For this review, take the finished solid that the model builds, in its own axes (mm). Face numbers are marked on the shaded views. Round coordinates to 2 decimals unless told otherwise and drop trailing zeros. Loops run counter-clockwise (first coordinate to the right, second up) from the corner with the lowest first, then second, coordinate; pieces in that order, holes last. Notation, with made-up numbers: (-10.5, 11) -> (6.5, 11) arc R17 ccw to (6.5, 24) -> close; hole circle Ø8 at (71.25, 10.25). An arc over 180 degrees is marked (long way). Use one line per item in the form item = value. Start each with the question number.
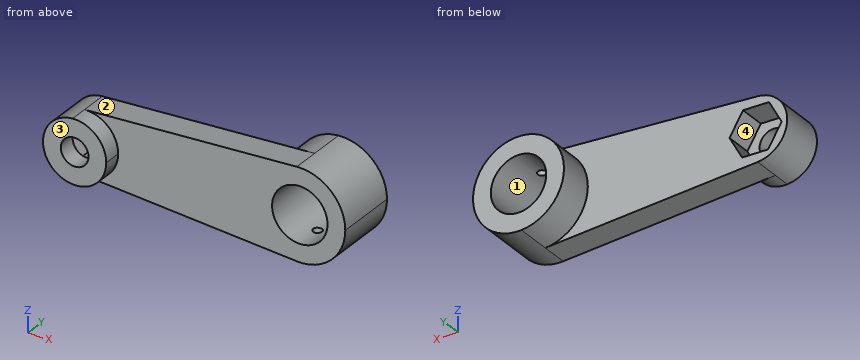
from build123d import *

# Parameters (mm, degrees)
F0_R     = 4.953
F1_DEPTH = 15.875
F0_R_2   = 9.906
F2_DEPTH = 9.525
F3_DEPTH = 12.7
F5_DEPTH = 9.525
F6_R     = 1.5875
F7_DEPTH = 15.875


with BuildPart() as f1:
    # F0 (on Front) → F1 (new body)
    with BuildSketch(Plane.XZ):
        with BuildLine():
            ThreePointArc((-0.734695, -11.279097), (7.72831, -8.248093), (11.303, 0))
            ThreePointArc((11.303, 0), (7.72831, 8.248093), (-0.734695, 11.279097))
            ThreePointArc((-0.734695, 11.279097), (-11.303, 0), (-0.734695, -11.279097))
        make_face()
        Circle(F0_R, mode=Mode.SUBTRACT)
    extrude(amount=F1_DEPTH)

    # F0 (on Front) → F2 (join)
    with BuildSketch(Plane.XZ):
        with BuildLine():
            ThreePointArc((-0.734695, -11.279097), (7.72831, -8.248093), (11.303, 0))
            ThreePointArc((11.303, 0), (7.72831, 8.248093), (-0.734695, 11.279097))
            ThreePointArc((-0.734695, 11.279097), (-11.303, 0), (-0.734695, -11.279097))
        make_face()
        Circle(F0_R, mode=Mode.SUBTRACT)
        with BuildLine():
            ThreePointArc((-0.734695, 11.279097), (7.72831, 8.248093), (11.303, 0))
            ThreePointArc((11.303, 0), (7.72831, -8.248093), (-0.734695, -11.279097))
            Line((-0.734695, -11.279097), (75.14336, -16.221623))
            ThreePointArc((75.14336, -16.221623), (59.944, 0), (75.14336, 16.221623))
            Line((75.14336, 16.221623), (-0.734695, 11.279097))
        make_face()
        with BuildLine():
            ThreePointArc((92.456, 0), (87.314873, 11.862425), (75.14336, 16.221623))
            ThreePointArc((75.14336, 16.221623), (59.944, 0), (75.14336, -16.221623))
            ThreePointArc((75.14336, -16.221623), (87.314873, -11.862425), (92.456, 0))
        make_face()
        with Locations((76.2, 0)):
            Circle(F0_R_2, mode=Mode.SUBTRACT)
    extrude(amount=F2_DEPTH)

    # F0 (on Front) → F3 (join)
    with BuildSketch(Plane.XZ):
        with BuildLine():
            ThreePointArc((92.456, 0), (87.314873, 11.862425), (75.14336, 16.221623))
            ThreePointArc((75.14336, 16.221623), (59.944, 0), (75.14336, -16.221623))
            ThreePointArc((75.14336, -16.221623), (87.314873, -11.862425), (92.456, 0))
        make_face()
        with Locations((76.2, 0)):
            Circle(F0_R_2, mode=Mode.SUBTRACT)
    extrude(amount=-F3_DEPTH)

    # F4 (on Front) → F5 (cut)
    with BuildSketch(Plane.XZ):
        Polygon((-4.819749, 7.967741), (-9.310141, -0.190155), (-4.490392, -8.157896), (4.819749, -7.967741), (9.310141, 0.190155), (4.490392, 8.157896), align=None)
    extrude(amount=F5_DEPTH, mode=Mode.SUBTRACT)

    # F6 (on Top) → F7 (cut, symmetric)
    with BuildSketch(Plane.XY):
        with Locations((76.223016, 0)):
            Circle(F6_R)
    extrude(amount=F7_DEPTH, both=True, mode=Mode.SUBTRACT)


solid = f1.part
Item 1: Take a section at B-B on y = -5.25. Give the boundary of the cut face in (x, z), plus the area to 3 significant figures.
Item 2: Draft analysis for pull direction Z (two halves, no side actions). For the marked faces 1, 2, 3 and 4, state which applies: +Z half, -Z half, draft (parallel to the pull), parting line (faces both ways), or undercut.
Item 3: For P1, Ø4, axis at x = 52, y = -6.5, coming from the +Z side; P2, Ø12, axis at x = 76.2, z = 0, coming from the +Y side; P3, Ø10, axis at y = -5, z = -10.5, coming from the +X side; P4, Ø1.5, axis at x = 7, y = -9, coming from the -Z side, all flat-tipped, find the tip position at first contact; note any pin that passes through.
Item 4: Wall thickness on line 1 (X direction, y = -1.75, z = -7); line 2 (Z direction, x = 0, y = -13.25); line 3 (X direction, y = -1.25, z = -1): over which ranges is each line inside the solid? List them lowest first.
Item 5: Take a section at D-D on z = -2. Give the boundary of the cut face in (x, y) (1 decimal).
Item 6: Take a section at A-A on x = 76.2. Give the boundary of the cut face in (y, z) (3 decimals).
Item 7: Take a section at C-C on z = 14.5. Give the boundary of the cut face in (x, y) (1 decimal), plus the area to 3 significant figures.
Results:
q1.outline = (-0.73, -11.28) -> (75.14, -16.22) arc R16.26 ccw to (92.46, 0) arc R16.26 ccw to (75.14, 16.22) -> (-0.73, 11.28) arc R11.3 ccw to start; hole (-9.31, -0.19) -> (-4.49, -8.16) -> (4.82, -7.97) -> (9.31, 0.19) -> (4.49, 8.16) -> (-4.82, 7.97) -> close; hole circle Ø19.81 at (76.2, 0)
q1.area = 2,190 mm2
q2.face_1 = undercut
q2.face_2 = +Z half
q2.face_3 = draft
q2.face_4 = undercut
q3.P1 = 14.84
q3.P2 = through
q3.P3 = 91.5
q3.P4 = -11.83
q4.line_1 = -8.87 to -5.19, 5.35 to 69.19, 83.21 to 90.87
q4.line_2 = -11.3 to -4.95, 4.95 to 11.3
q4.line_3 = -11.26 to -8.82, 8.66 to 66.34, 86.06 to 92.43
q5.outline = (-11.1, -15.9) -> (-4.5, -15.9) -> (-4.5, -9.5) -> (-8.2, -9.5) -> (-8.2, 0) -> (-11.1, 0) -> close; (4.5, -15.9) -> (11.1, -15.9) -> (11.1, -9.5) -> (66.5, -9.5) -> (66.5, 12.7) -> (60.1, 12.7) -> (60.1, 0) -> (8.1, 0) -> (8.1, -9.5) -> (4.5, -9.5) -> close; (85.9, -9.5) -> (92.3, -9.5) -> (92.3, 12.7) -> (85.9, 12.7) -> close
q6.outline = (-9.525, -16.256) -> (12.7, -16.256) -> (12.7, -9.906) -> (1.587, -9.906) -> (1.587, -15.875) -> (-1.587, -15.875) -> (-1.587, -9.906) -> (-9.525, -9.906) -> close; (-9.525, 9.906) -> (-1.587, 9.906) -> (-1.587, 15.875) -> (1.587, 15.875) -> (1.587, 9.906) -> (12.7, 9.906) -> (12.7, 16.256) -> (-9.525, 16.256) -> close
q7.outline = (48.7, -9.5) -> (83.5, -9.5) -> (83.5, 12.7) -> (68.9, 12.7) -> (68.9, 0) -> (48.7, 0) -> close; hole circle Ø3.2 at (76.2, 0)
q7.area = 511 mm2
